from build123d import *

# Parameters (mm, degrees)
F0_W     = 195
F0_H     = 195
F1_DEPTH = 170
F3_R     = 25
F4_T     = -30
F2_R     = 4.5
F5_DEPTH = 195
F6_DEPTH = 40


with BuildPart() as f1:
    # F0 (on Top) → F1 (new body)
    with BuildSketch(Plane.XY):
        Rectangle(F0_W, F0_H)
    extrude(amount=F1_DEPTH)

    # F3
    f3_edges = [f1.edges().sort_by_distance(p)[0] for p in [
        (97.5, 0, 0),
        (0, 97.5, 0),
        (-97.5, 0, 0),
        (0, -97.5, 0),
        (97.5, 97.5, 85),
        (-97.5, 97.5, 85),
        (-97.5, -97.5, 85),
        (97.5, -97.5, 85),
    ]]
    fillet(f3_edges, radius=F3_R)

    # F4
    f4_openings = [f1.faces().sort_by_distance(p)[0] for p in [
        (0, 0, 170),
    ]]
    offset(amount=F4_T, openings=f4_openings)

    # F2 (on Right) → F5 (cut)
    with BuildSketch(Plane.YZ):
        with Locations((-25, 12.5)):
            Circle(F2_R)
        with Locations((25, 12.5)):
            Circle(F2_R)
    extrude(amount=-F5_DEPTH, mode=Mode.SUBTRACT)

    # F2 (on Right) → F6 (cut)
    with BuildSketch(Plane.YZ):
        with Locations((-25, 12.5)):
            Circle(F2_R)
        with Locations((25, 12.5)):
            Circle(F2_R)
    extrude(amount=F6_DEPTH, mode=Mode.SUBTRACT)


solid = f1.part
Verification items for the finished model (mm, model axes). A direction names the side the tool comes from. Coordinates: 2 decimals unless noted, no trailing zeros. Order: outer loops, then holes, each group sorted by start corner. A loop starts at its lowest first (then second) coordinate and runs counter-clockwise, first axis right, second up. Notation, with made-up numbers: M -28.5,77.25 L -10.5,77.25 A33 ccw -10.5,114.25 Z; hole C 0,64.25 d4. An arc over 180 degrees is marked long. One line per item, written item: value. Start each with the question number.
Item 1: Sectioned sample at B-B (x = -18.5). Enter the section's corners in (y, z).
Item 2: Scan lines: probe 1 along X at (y, z) = (38, 102); probe 2 along Y at (x, z) = (-27, 12.5); probe 3 along Z at (x, y) = (-56.5, 55). Record each from-to range of solid material in increasing order.
Item 3: Gauge pin test, flat ends, axial feed: pin 1 (3 mm diameter, centred on x = 31.5, y = 52.5, fed in from +Z); pin 2 (8 mm diameter, centred on y = -25, z = 12.5, fed in from -X); pin 3 (11.5 mm diameter, centred on y = 25, z = 12.5, fed in from +X). Record the tip position at first contact, or that the pin passes through.
Item 4: Mould release check, pull along X, two halves, no side actions. Record for faces 1 (the flat face through (-1, -67.5, 99)), 2 (the cylindrical face through (1.015, 90.371, 7.518)), 3 (the cylindrical face through (90.371, 89.982, 98.515)): released by +X, released by -X, zero draft, split by the parting line, or undercut.
Item 5: Access from +Z, -Z, +X, -X, +Y, -Y to the whole of each face (thin tool, end or side, straight path). Record for faces 4 (the flat face through (-1, 67.5, 99)), 5 (the flat face through (97.5, -1, 96)), 6 (the flat face through (40, 25, 13)).
Item 6: Sectioned sample at A-A (z = 79.5). Enter the section's corners in (x, y), then the cut area to 3 significant figures.
Item 7: Sectioned sample at C-C (y = -2). Enter the section's corners in (x, z).
Conclusion:
1. outline: M -97.5,25 A25 ccw -72.5,0 L 72.5,0 A25 ccw 97.5,25 L 97.5,170 L 67.5,170 L 67.5,30 L -67.5,30 L -67.5,170 L -97.5,170 Z; hole C -25,12.5 d9; hole C 25,12.5 d9
2. probe 1: x = -97.5 to -67.5, 67.5 to 97.5
2. probe 2: y = -94.15 to -29.5, -20.5 to 20.5, 29.5 to 94.15
2. probe 3: z = 0 to 30
3. pin 1: stops at z = 30
3. pin 2: stops at x = 40
3. pin 3: stops at x = 96.57
4. face 1: undercut
4. face 2: zero draft
4. face 3: released by +X
5. face 4: +Z
5. face 5: +Z, -Z, +X, +Y, -Y
5. face 6: -X
6. outline: M -97.5,-72.5 A25 ccw -72.5,-97.5 L 72.5,-97.5 A25 ccw 97.5,-72.5 L 97.5,72.5 A25 ccw 72.5,97.5 L -72.5,97.5 A25 ccw -97.5,72.5 Z; hole M -67.5,-67.5 L 67.5,-67.5 L 67.5,67.5 L -67.5,67.5 Z
6. area: 19,300 mm^2
7. outline: M -97.5,25 A25 ccw -72.5,0 L 72.5,0 A25 ccw 97.5,25 L 97.5,170 L 67.5,170 L 67.5,30 L -67.5,30 L -67.5,170 L -97.5,170 Z
